from build123d import *

# Parameters (mm, degrees)
SKETCH1_W                  = 304.8
SKETCH1_H                  = 9.525
BOSS_EXTRUDE1_DEPTH        = 31.75
F_10_24_TAPPED_HOLE1_D     = 3.7973
F_10_24_TAPPED_HOLE1_DEPTH = 19.05
F_10_24_TAPPED_HOLE1_TIP   = 1.140824014
FILLET1_R                  = 1.27


with BuildPart() as part:
    # Sketch1 → Boss-Extrude1 (new body)
    with BuildSketch(Plane(origin=(0, -21, 0), x_dir=(1, 0, 0), z_dir=(0, 1, 0))):
        with Locations((6.69e-07, -174.7625)):
            Rectangle(SKETCH1_W, SKETCH1_H)
    extrude(amount=BOSS_EXTRUDE1_DEPTH)

    # #10-24 Tapped Hole1
    with Locations(Plane(origin=(0, -21, 0), x_dir=(-1, 0, 0), z_dir=(0, -1, 0))):
        with Locations((-127.000000669, -174.7625), (-42.333334002, -174.7625), (126.999999331, -174.7625), (42.333332664, -174.7625)):
            Hole(F_10_24_TAPPED_HOLE1_D / 2, depth=F_10_24_TAPPED_HOLE1_DEPTH)
            with Locations((0, 0, -(F_10_24_TAPPED_HOLE1_DEPTH + F_10_24_TAPPED_HOLE1_TIP / 2))):  # 118° drill point
                Cone(0, F_10_24_TAPPED_HOLE1_D / 2, F_10_24_TAPPED_HOLE1_TIP, mode=Mode.SUBTRACT)

    # Sketch5 → #10-24 Tapped Hole2 (revolve, cut)
    with BuildSketch(Plane(origin=(152.400000669, -5.125, 174.7625), x_dir=(0, 0, -1), z_dir=(0, 1, 0))):
        Polygon((0, 0), (0, 20.190824014), (1.89865, 19.05), (1.89865, 0), align=None)
    f_10_24_tapped_hole2 = revolve(axis=Axis((158.750000669, -5.125, 174.7625), (-1, 0, 0)), mode=Mode.SUBTRACT)

    # Mirror1: #10-24 Tapped Hole2 across plane
    add(f_10_24_tapped_hole2.mirror(Plane(origin=(0, 0, 0), x_dir=(0, 0, 1), z_dir=(1, 0, 0))), mode=Mode.SUBTRACT)

    # Fillet1
    fillet1_edges = [part.edges().sort_by_distance(p)[0] for p in [
        (152.400000669, -5.125, 170),
        (152.400000669, -5.125, 179.525),
        (-152.399999331, -5.125, 179.525),
        (-152.399999331, -5.125, 170),
    ]]
    fillet(fillet1_edges, radius=FILLET1_R)


solid = part.part
Input: part model. Units: mm. Frame: model coordinates. Give positions to 0.01 mm unless a question says otherwise; leave off trailing zeros. Order: outer loops, then holes, each group sorted by start corner. A loop starts at its lowest first (then second) coordinate and runs counter-clockwise, first axis right, second up. Notation, with made-up numbers: M -4.5,75 L 4.5,75 A22 cw 4.5,107 Z; hole C 77.25,52.5 d10. An arc over 180 degrees is marked long. Answer as a JSON object with one key per item and string values.
1. Ray query, line 1 (Z direction, x = -127, y = -15.75) (3 decimals); line 2 (X direction, y = -8, z = 173.5); line 3 (X direction, y = -8.5, z = 175.5). Return the intervals inside material, ascending. Write a range as [from, to].
Result sheet:
{"line 1": "[170, 172.864], [176.661, 179.525]", "line 2": "[-152.4, -128.42], [-125.58, -43.75], [-40.92, 40.92], [43.75, 125.58], [128.42, 152.4]", "line 3": "[-152.4, -128.75], [-125.25, -44.08], [-40.58, 40.58], [44.08, 125.25], [128.75, 152.4]"}
2. Cut plane A-A, the plane y = -17. Output: boundary loops of the cut face in (x, z) (1 decimal).
Result sheet:
{"outline": "M -152.4,171.3 A1.3 ccw -151.1,170 L 151.1,170 A1.3 ccw 152.4,171.3 L 152.4,178.3 A1.3 ccw 151.1,179.5 L -151.1,179.5 A1.3 ccw -152.4,178.3 Z; hole C -127,174.8 d3.8; hole C -42.3,174.8 d3.8; hole C 42.3,174.8 d3.8; hole C 127,174.8 d3.8"}
3. First-contact query: P1, Ø3, axis at y = -5.12, z = 174.76, coming from the +X side; P2, Ø2.5, axis at x = 42.33, z = 174.76, coming from the -Y side. Flat tips, straight axial feed; report the tip coordinate or a pass-through.
Result sheet:
{"P1": "x = 133.11", "P2": "y = -1.56"}
